from build123d import *

# Parameters (mm, degrees)
EXTRUDE1_DEPTH     = 15
EXTRUDE2_DEPTH     = 70
CUT_EXTRUDE1_DEPTH = 60


with BuildPart() as part:
    # Sketch1 → Extrude1 (new body)
    with BuildSketch(Plane(origin=(0, 0, 0), x_dir=(1, 0, 0), z_dir=(0, 1, 0))):
        Polygon((-58.97114317, 12.141016151), (18.97114317, 57.141016151), (58.97114317, -12.141016151), (-18.97114317, -57.141016151), align=None)
    extrude(amount=EXTRUDE1_DEPTH)

    # Sketch2 → Extrude2 (add)
    with BuildSketch(Plane(origin=(0, 15, 0), x_dir=(-1, 0, 0), z_dir=(0, 1, 0))):
        Polygon((38.480762114, -6.650635095), (-13.480762114, -36.650635095), (-38.480762114, 6.650635095), (13.480762114, 36.650635095), align=None)
    extrude(amount=EXTRUDE2_DEPTH)

    # Sketch3 → Cut-Extrude1 (cut)
    with BuildSketch(Plane(origin=(-25.980762114, 0, 15), x_dir=(0.5, 0, 0.866025404), z_dir=(-0.866025404, 0, 0.5))):
        Polygon((-25, 15), (-25, 85), (-10, 50), align=None)
        Polygon((25, 85), (25, 15), (10, 50), align=None)
    extrude(amount=-CUT_EXTRUDE1_DEPTH, mode=Mode.SUBTRACT)

    # Sketch4 → Loft1 section 0
    with BuildSketch(Plane(origin=(0, 85, 0), x_dir=(-1, 0, 0), z_dir=(0, 1, 0)), mode=Mode.PRIVATE) as loft1_s0:
        Polygon((38.480762114, -6.650635095), (-13.480762114, -36.650635095), (-38.480762114, 6.650635095), (13.480762114, 36.650635095), align=None)
    loft([loft1_s0.sketch, Vertex(0, 110, 0)])


solid = part.part
Part model, mm, in its own coordinate system. A direction names the side the tool comes from. Coordinates: 2 decimals unless noted, no trailing zeros. Write each loop counter-clockwise with the first axis right and the second up, starting at its lowest first coordinate (ties: lowest second). Pieces come first, ordered by that corner, then holes. Notation, with made-up numbers: M -29,61 L -12,61 A16 ccw -12,72 Z; hole C 30,16 d3. An arc over 180 degrees is marked long. Return JSON: item names as keys, results as strings.
1. Saw through at C-C, the plane x = 9. Write the cut outline in (y, z).
Determined:
{"outline": "M 0,-51.38 L 15,-51.38 L 15,-34.06 L 50,-16.74 L 85,-34.06 L 93.31,-24.47 L 104.15,1.56 L 85,23.67 L 50,6.35 L 15,23.67 L 15,40.99 L 0,40.99 Z"}
2. Pull direction Y, two halves, no side cores. Call faces 4 (the face through (7.915, 94.897, 12.869)), 5 (the face through (-9.166, 67.745, -15.036)), 6 (the face through (20.546, 7.395, 34.326)): pulls with the +Y half, pulls with the -Y half, needs draft (parallel to the pull), parting line crosses it, or undercut.
Determined:
{"face 4": "pulls with the +Y half", "face 5": "undercut", "face 6": "needs draft"}
3. Saw through at A-A, the plane z = 34. Write the cut outline in (x, y).
Determined:
{"outline": "M -32.33,0 L 21.11,0 L 21.11,15 L -8.89,15 L -15.01,22.14 L -15.01,15 L -32.33,15 Z; M -15.01,77.86 L -8.89,85 L -12.51,86.81 L -15.01,85 Z"}
4. Saw through at D-D, the plane y = 78.5. Write the cut outline in (x, z).
Determined:
{"outline": "M -37.09,-4.24 L 14.87,-34.24 L 37.09,4.24 L -14.87,34.24 Z"}
5. 3-axis set-ups, long thin cutter, end or side, ignore diameter. For faces 1 (the face through (8.334, 67.255, 15.275)), 2 (the face through (25.806, 49.51, -15.303)), 3 (the face through (-22, 15, -17)): which of +Z, -Z, +X, -X, +Y, -Y reach the whole face in a straight line?
Determined:
{"face 1": "+Z, +X", "face 2": "-Z, +X, +Y", "face 3": "+Y"}
6. Probe L1, parallel to Y at x = -17, z = -36; L2, parallel to Y at x = -5, z = 27; L3, parallel to Z at x = -4.5, y = 104. List the from-to ranges inside material, lowest first.
Determined:
{"L1": "0 to 15", "L2": "0 to 24.61, 75.39 to 89.12", "L3": "-4.33 to 6.61"}
7. Flat gauge pins, fed straight in: pin 1 Ø12 at (y, z) = (87, -39.5) entering from +X; pin 2 Ø10 at (y, z) = (66.5, -20) entering from +X; pin 3 Ø1.5 at (y, z) = (12.5, 15.5) entering from -X; pin 4 Ø6 at (y, z) = (93, -33) entering from -X. Where does each tip first touch, or does it go through?
Determined:
{"pin 1": "x = 15.1", "pin 2": "x = 25.98", "pin 3": "x = -43.45", "pin 4": "through"}
8. Saw through at B-B, the plane z = 21. Write the cut outline in (x, y), then the cut area to 3 significant figures.
Determined:
{"outline": "M -39.84,0 L 43.63,0 L 43.63,15 L 13.63,15 L -16.37,50 L 13.63,85 L -7.72,95.68 L -22.52,85 L -22.52,15 L -39.84,15 Z", "area": "2,920 mm²"}
